Geometry: final body of the model. Coordinates: model frame, mm. A direction names the side the tool comes from. Give positions to 0.01 mm unless a question says otherwise; leave off trailing zeros. Order: outer loops, then holes, each group sorted by start corner. A loop starts at its lowest first (then second) coordinate and runs counter-clockwise, first axis right, second up. Notation, with made-up numbers: (86.25, -2) -> (129.25, -2) arc R22 ccw to (129.25, 7) -> close; hole circle Ø6 at (52, 18.25). An arc over 180 degrees is marked (long way). Answer in a Markdown table with one row per item. Add a question column.
Q1. Cut plane A-A on z = 38. Return the cut outline in (x, y).
Q2. Cut plane B-B on y = 18. Return the cut outline in (x, z), and give its area (3 significant figures).
Q3. Set-up query: faces 4 (the face through (253.859, 1, 74)), 5 (the face through (0, -67.849, 79)). Return all of +Z, -Z, +X, -X, +Y, -Y with unobstructed straight access to the full face (end or side cutting, diameter ignored); none if empty.
Q4. Line query: line 1 along Y through (x, z) = (215.5, 34); line 2 along X through (y, z) = (55.5, 50.5); line 3 along Z through (x, y) = (-149, 27.5). Output: solid intervals per line, ascending. Write a range as from..to.
Q5. Cut plane C-C on x = 3.5. Return the cut outline in (y, z).
Q6. Contact query for a flat-ended pin moving along its axis: P1, Ø2, axis at x = -27, y = -39, coming from the +Z side. Output: stop coordinate, or through.
Q7. Pull-direction query (Y, two-part tool) for faces 1 (the face through (0, 3, 0)), 2 (the face through (-241.7, -68.29, 73.95)), 3 (the face through (-241.141, 1, 79)); classes: +Y half, -Y half, draft (parallel to the pull), parting line (faces both ways), or undercut.
from build123d import *

# Parameters (mm, degrees)
F0_W     = 500
F0_H     = 150
F1_DEPTH = 150
F2_W     = 490
F2_H     = 140
F3_DEPTH = 145
F4_SIZE  = 9
F5_SIZE  = 9


with BuildPart() as f1:
    # F0 (on Top) → F1 (new body)
    with BuildSketch(Plane.XY):
        with Locations((3.85901, 2.15064)):
            Rectangle(F0_W, F0_H)
    extrude(amount=F1_DEPTH)

    # F2 (on face) → F3 (cut)
    with BuildSketch(Plane.XY.offset(150)):
        with Locations((3.85901, 2.15064)):
            Rectangle(F2_W, F2_H)
    extrude(amount=-F3_DEPTH, mode=Mode.SUBTRACT)

    # F4
    f4_edges = [f1.edges().sort_by_distance(p)[0] for p in [
        (253.85901, -72.84936, 75),
    ]]
    chamfer(f4_edges, length=F4_SIZE)

    # F5
    f5_edges = [f1.edges().sort_by_distance(p)[0] for p in [
        (253.85901, 77.15064, 75),
        (-246.14099, 77.15064, 75),
        (-246.14099, -72.84936, 75),
    ]]
    chamfer(f5_edges, length=F5_SIZE)


solid = f1.part
Completed:
| question | item | result |
|---|---|---|
| 1 | outline | (-246.14, -63.85) -> (-237.14, -72.85) -> (244.86, -72.85) -> (253.86, -63.85) -> (253.86, 68.15) -> (244.86, 77.15) -> (-237.14, 77.15) -> (-246.14, 68.15) -> close; hole (-241.14, -67.85) -> (248.86, -67.85) -> (248.86, 72.15) -> (-241.14, 72.15) -> close |
| 2 | outline | (-246.14, 0) -> (253.86, 0) -> (253.86, 150) -> (248.86, 150) -> (248.86, 5) -> (-241.14, 5) -> (-241.14, 150) -> (-246.14, 150) -> close |
| 2 | area | 3,950 mm² |
| 3 | face 4 | +Z, -Z, +X, +Y, -Y |
| 3 | face 5 | +Z |
| 4 | line 1 | y = -72.85..-67.85, 72.15..77.15 |
| 4 | line 2 | x = -246.14..-241.14, 248.86..253.86 |
| 4 | line 3 | z = 0..5 |
| 5 | outline | (-72.85, 0) -> (77.15, 0) -> (77.15, 150) -> (72.15, 150) -> (72.15, 5) -> (-67.85, 5) -> (-67.85, 150) -> (-72.85, 150) -> close |
| 6 | P1 | stops at z = 5 |
| 7 | face 1 | draft |
| 7 | face 2 | -Y half |
| 7 | face 3 | undercut |
